from build123d import *

# Parameters (mm, degrees)
ESQUISSE1_W             = 200
ESQUISSE1_H             = 100
BOSS_EXTRU_1_DEPTH      = 10
ESQUISSE2_W             = 10
ESQUISSE2_H             = 25
BOSS_EXTRU_2_DEPTH      = 10
ESQUISSE3_R             = 1.5
ENL_V_MAT_EXTRU_1_DEPTH = 201


with BuildPart() as part:
    # Esquisse1 → Boss.-Extru.1 (new body)
    with BuildSketch(Plane.XY):
        with Locations((-100, 50)):
            Rectangle(ESQUISSE1_W, ESQUISSE1_H)
    extrude(amount=BOSS_EXTRU_1_DEPTH)

    # Esquisse2 → Boss.-Extru.2 (add)
    with BuildSketch(Plane.XY.offset(10)):
        with Locations((-195, 50)):
            Rectangle(ESQUISSE2_W, ESQUISSE2_H)
        with Locations((-5, 50)):
            Rectangle(ESQUISSE2_W, ESQUISSE2_H)
    extrude(amount=BOSS_EXTRU_2_DEPTH)

    # Esquisse3 → Enlèv. mat.-Extru.1 (cut, through all)
    with BuildSketch(Plane.ZY.offset(200)):
        with Locations((15, 50)):
            Circle(ESQUISSE3_R)
    extrude(amount=-ENL_V_MAT_EXTRU_1_DEPTH, mode=Mode.SUBTRACT)


solid = part.part
Design review of the part built by this model. Coordinates are the model's own, in mm. A direction names the side the tool comes from. Coordinates: 2 decimals unless noted, no trailing zeros. Order: outer loops, then holes, each group sorted by start corner. A loop starts at its lowest first (then second) coordinate and runs counter-clockwise, first axis right, second up. Notation, with made-up numbers: (-22.75, -30.5) -> (22.25, -30.5) arc R21 ccw to (22.25, -18.5) -> close; hole circle Ø9 at (8, 82). An arc over 180 degrees is marked (long way). Use one line per item in the form item = value. Start each with the question number.
(1) Add section A-A on y = 45.5. State the section outline as (x, z) points, plus the area to 3 significant figures.
(2) Add section B-B on x = -98. State the section outline as (y, z) points.
(3) For faces 1 (the flat face through (-195, 62.5, 15)), 2 (the flat face through (-101, 100, 5)), 3 (the flat face through (-5, 37.5, 15)), 4 (the flat face through (-5, 50, 20)), 5 (the flat face through (-190, 50, 17)), list the 3-axis set-ups (+Z, -Z, +X, -X, +Y, -Y) from which the entire face can be reached by the end or side of a thin tool; tool diameter is ignored.
(4) Insertion check: pin 1 (4 mm diameter, centred on x = -125.5, y = 21, fed in from +Z); pin 2 (11 mm diameter, centred on x = -6, z = 17, fed in from +Y); pin 3 (3 mm diameter, centred on x = -3.5, z = 17, fed in from -Y). Each pin has a flat end and moves straight along its axis. Give the tip position at first contact, or say it passes through.
(5) Add section C-C on y = 81.5. State the section outline as (x, z) points.
(6) The part is to be moulded in two halves that separate along X. For faces 6 (the flat face through (0, 49, 8)), 7 (the flat face through (-200, 49, 8)), 8 (the flat face through (-10, 50, 17)), say which applies: +X half, -X half, draft (parallel to the pull), parting line (faces both ways), or undercut.
(7) For probe 1 along Y at (x, z) = (-194.25, 15); probe 2 along X at (y, z) = (54, 14); probe 3 along Z at (x, y) = (-91, 79), list the stretches that pass through material, from the lowest coordinate up.
Answer block:
q1.outline = (-200, 0) -> (0, 0) -> (0, 20) -> (-10, 20) -> (-10, 10) -> (-190, 10) -> (-190, 20) -> (-200, 20) -> close
q1.area = 2,200 mm²
q2.outline = (0, 0) -> (100, 0) -> (100, 10) -> (0, 10) -> close
q3.face_1 = +Z, +X, -X, +Y
q3.face_2 = +Z, -Z, +X, -X, +Y
q3.face_3 = +Z, +X, -X, -Y
q3.face_4 = +Z, +X, -X, +Y, -Y
q3.face_5 = +Z, +Y, -Y
q4.pin_1 = 10
q4.pin_2 = 62.5
q4.pin_3 = 37.5
q5.outline = (-200, 0) -> (0, 0) -> (0, 10) -> (-200, 10) -> close
q6.face_6 = +X half
q6.face_7 = -X half
q6.face_8 = undercut
q7.probe_1 = 37.5 to 48.5, 51.5 to 62.5
q7.probe_2 = -200 to -190, -10 to 0
q7.probe_3 = 0 to 10
